```python
from build123d import *

# Parameters (mm, degrees)
SKETCH_1_R      = 3
SKETCH_1_R_2    = 1.25
SKETCH_1_R_3    = 1
EXTRUDE_2_DEPTH = 2


with BuildPart() as part:
    # 草圖1 → 填料-伸長2 (new body)
    with BuildSketch(Plane.XY):
        with BuildLine():
            Line((-7.587453917, -13.1179941), (18.058094933, -13.1179941))
            Line((18.058094933, -13.1179941), (19.058094933, -13.1179941))
            Line((19.058094933, -13.1179941), (19.058094933, -12.1179941))
            Line((19.058094933, -12.1179941), (19.058094933, -2.1179941))
            ThreePointArc((19.058094933, -2.1179941), (18.058094933, -1.1179941), (19.058094933, -0.1179941))
            Line((19.058094933, -0.1179941), (21.058094933, -0.1179941))
            Line((21.058094933, -0.1179941), (21.058094933, 3.8820059))
            Line((21.058094933, 3.8820059), (19.058094933, 3.8820059))
            ThreePointArc((19.058094933, 3.8820059), (18.058094933, 4.8820059), (19.058094933, 5.8820059))
            Line((19.058094933, 5.8820059), (19.058094933, 9.8820059))
            Line((19.058094933, 9.8820059), (19.058094933, 10.8820059))
            Line((19.058094933, 10.8820059), (19.058094933, 16.8820059))
            Line((19.058094933, 16.8820059), (19.058094933, 17.8820059))
            Line((19.058094933, 17.8820059), (18.058094933, 17.8820059))
            Line((18.058094933, 17.8820059), (-27.541905067, 17.8820059))
            Line((-27.541905067, 17.8820059), (-28.541905067, 17.8820059))
            Line((-28.541905067, 17.8820059), (-28.541905067, 16.8820059))
            Line((-28.541905067, 16.8820059), (-28.541905067, 10.8820059))
            Line((-28.541905067, 10.8820059), (-28.541905067, 9.8820059))
            Line((-28.541905067, 9.8820059), (-28.541905067, 5.8820059))
            ThreePointArc((-28.541905067, 5.8820059), (-27.541905067, 4.8820059), (-28.541905067, 3.8820059))
            Line((-28.541905067, 3.8820059), (-30.541905067, 3.8820059))
            Line((-30.541905067, 3.8820059), (-30.541905067, -0.1179941))
            Line((-30.541905067, -0.1179941), (-28.541905067, -0.1179941))
            ThreePointArc((-28.541905067, -0.1179941), (-27.541905067, -1.1179941), (-28.541905067, -2.1179941))
            Line((-28.541905067, -2.1179941), (-28.541905067, -13.1179941))
            ThreePointArc((-28.541905067, -13.1179941), (-18.541905067, -23.1179941), (-8.541905067, -13.1179941))
            Line((-8.541905067, -13.1179941), (-7.587453917, -13.1179941))
        make_face()
        with Locations((-18.541905067, -13.1179941)):
            Circle(SKETCH_1_R, mode=Mode.SUBTRACT)
        with Locations((-18.541905067, -6.1179941)):
            Circle(SKETCH_1_R_2, mode=Mode.SUBTRACT)
        with Locations((-13.592157599, -8.168246632)):
            Circle(SKETCH_1_R_2, mode=Mode.SUBTRACT)
        with Locations((-11.541905067, -13.1179941)):
            Circle(SKETCH_1_R_2, mode=Mode.SUBTRACT)
        with Locations((-13.592157599, -18.067741569)):
            Circle(SKETCH_1_R_2, mode=Mode.SUBTRACT)
        with Locations((-18.541905067, -20.1179941)):
            Circle(SKETCH_1_R_2, mode=Mode.SUBTRACT)
        with Locations((-23.491652536, -18.067741569)):
            Circle(SKETCH_1_R_2, mode=Mode.SUBTRACT)
        with Locations((-25.541905067, -13.1179941)):
            Circle(SKETCH_1_R_2, mode=Mode.SUBTRACT)
        with Locations((-23.491652536, -8.168246632)):
            Circle(SKETCH_1_R_2, mode=Mode.SUBTRACT)
        with Locations((-26.541905067, 1.8820059)):
            Circle(SKETCH_1_R_3, mode=Mode.SUBTRACT)
        with Locations((17.058094933, 1.8820059)):
            Circle(SKETCH_1_R_3, mode=Mode.SUBTRACT)
        with Locations((-4.741905067, 13.8820059)):
            Circle(SKETCH_1_R_3, mode=Mode.SUBTRACT)
        with Locations((11.058094933, -5.1179941)):
            Circle(SKETCH_1_R_2, mode=Mode.SUBTRACT)
        with Locations((-16.741905067, 13.8820059)):
            Circle(SKETCH_1_R_3, mode=Mode.SUBTRACT)
        with Locations((7.258094933, 13.8820059)):
            Circle(SKETCH_1_R_3, mode=Mode.SUBTRACT)
    extrude(amount=EXTRUDE_2_DEPTH)


solid = part.part
```
Source: CAD feature listing. Evaluate the final solid. Frame: model axes, mm. A direction names the side the tool comes from. Round coordinates to 2 decimals unless told otherwise and drop trailing zeros. Loops run counter-clockwise (first coordinate to the right, second up) from the corner with the lowest first, then second, coordinate; pieces in that order, holes last.
1. Section query C-C on z = 1.2. Give the number of separate pieces and of enclosed holes in the cut face, and give its area (3 significant figures).
2. Section query A-A on y = -15.5. Output: boundary loops of the cut face in (x, z), and give its area (3 significant figures).
3. Section query B-B on x = -21. Output: boundary loops of the cut face in (y, z), and give its area (3 significant figures).
4. Section query D-D on x = 2.5. Output: boundary loops of the cut face in (y, z), and give its area (3 significant figures).
5. Ray query, L1, parallel to X at y = 2, z = 0.7; L2, parallel to Y at x = 17, z = 0.2; L3, parallel to X at y = 2.5, z = 0.7. Return the intervals inside material, ascending.
6. Mould query, pull axis X, two halves, no side actions, for faces 1 (the cylindrical face through (-4.872, 14.873, 0.986)), 2 (the cylindrical face through (18.06, -1.14, 0.99)), 3 (the flat face through (5, -13.118, 1)). Classes: released by +X, released by -X, zero draft, split by the parting line, or undercut.
7. Access query for faces 4 (the flat face through (19.058, -8, 1)), 5 (the flat face through (20, 3.882, 1)), 6 (the cylindrical face through (-27.54, 1.93, 0.99)), 7 (the flat face through (-28.542, -8, 1)), 8 (the flat face through (-28.542, 12, 1)). Directions: +Z, -Z, +X, -X, +Y, -Y. A direction counts if a zero-diameter tool reaches every point of the face in a straight line with its end or side. Return the directions, or none.
8. Contact query for flat-ended pins moving along their axis: pin 1 (1 mm diameter, centred on y = -8, z = 1, fed in from +X); pin 2 (1 mm diameter, centred on x = 8.5, z = 1, fed in from -Y); pin 3 (1 mm diameter, centred on x = 20, z = 1.5, fed in from -Y). Output: stop coordinate, or through.
Answers below:
1. separate pieces: 1
1. enclosed holes: 15
1. area: 1,550 mm2
2. outline: (-28.25, 0) - (-20.37, 0) - (-20.37, 2) - (-28.25, 2) - close; (-16.72, 0) - (-8.83, 0) - (-8.83, 2) - (-16.72, 2) - close
2. area: 31.6 mm2
3. outline: (-22.81, 0) - (-14.84, 0) - (-14.84, 2) - (-22.81, 2) - close; (-11.4, 0) - (17.88, 0) - (17.88, 2) - (-11.4, 2) - close
3. area: 74.5 mm2
4. outline: (-13.12, 0) - (17.88, 0) - (17.88, 2) - (-13.12, 2) - close
4. area: 62.0 mm2
5. L1: x = -30.54 to -27.53, -25.55 to 16.07, 18.05 to 21.06
5. L2: y = -13.12 to 0.88, 2.88 to 17.88
5. L3: x = -30.54 to -27.33, -25.76 to 16.27, 17.84 to 21.06
6. face 1: undercut
6. face 2: released by +X
6. face 3: zero draft
7. face 4: +Z, -Z, +X, -Y
7. face 5: +Z, -Z, +X, +Y
7. face 6: +Z, -Z
7. face 7: +Z, -Z, -X, -Y
7. face 8: +Z, -Z, -X, +Y
8. pin 1: stops at x = 19.06
8. pin 2: stops at y = -13.12
8. pin 3: stops at y = -0.12
